Part print with two shaded views. Sizes in mm from the minimum x, y, z corner. Give positions to 0.01 mm unless a question says otherwise; leave off trailing zeros. Write each loop counter-clockwise with the first axis right and the second up, starting at its lowest first coordinate (ties: lowest second). Pieces come first, ordered by that corner, then holes. Notation, with made-up numbers: (-16.75, 46) -> (-6.75, 46) arc R27 cw to (-6.75, 64) -> close; hole circle Ø2 at (64, 45). An arc over 180 degrees is marked (long way). Answer as a JSON object with one key per item and string values.
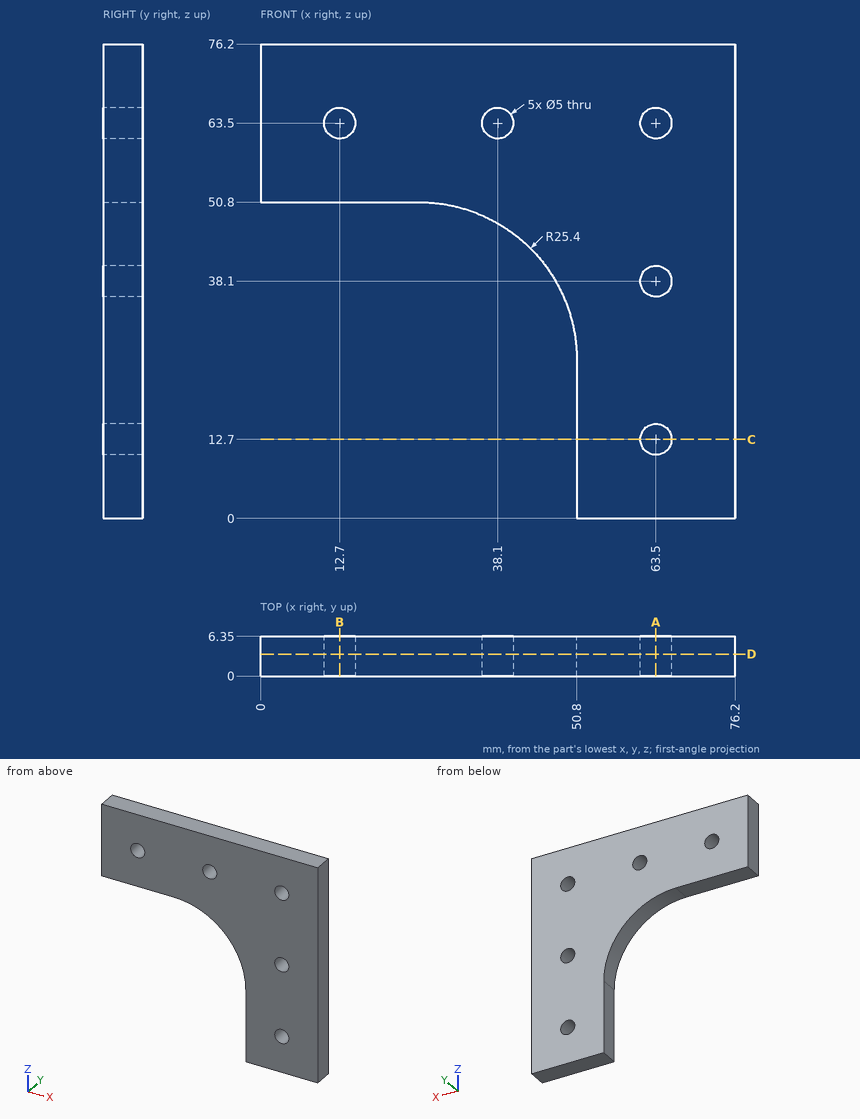
1) Slice it at B-B (x = 12.7). List the corners of the cut face in (y, z).
Model answer:
{"outline": "(0, 50.8) -> (6.35, 50.8) -> (6.35, 61) -> (0, 61) -> close; (0, 66) -> (6.35, 66) -> (6.35, 76.2) -> (0, 76.2) -> close"}
2) Slice it at D-D (y = 3.5). List the corners of the cut face in (x, z), then the cut area to 3 significant figures.
Model answer:
{"outline": "(0, 50.8) -> (25.4, 50.8) arc R25.4 cw to (50.8, 25.4) -> (50.8, 0) -> (76.2, 0) -> (76.2, 76.2) -> (0, 76.2) -> close; hole circle Ø5 at (12.7, 63.5); hole circle Ø5 at (38.1, 63.5); hole circle Ø5 at (63.5, 12.7); hole circle Ø5 at (63.5, 38.1); hole circle Ø5 at (63.5, 63.5)", "area": "3,270 mm2"}
3) Wall check: probe 1 along Z at (x, y) = (63.5, 3.25); probe 2 along Z at (x, y) = (12.7, 2.25); probe 3 along X at (y, z) = (5, 64.5). Give the ranges that are in metal, low to high.
Model answer:
{"probe 1": "z = 0 to 10.2, 15.2 to 35.6, 40.6 to 61, 66 to 76.2", "probe 2": "z = 50.8 to 61, 66 to 76.2", "probe 3": "x = 0 to 10.41, 14.99 to 35.81, 40.39 to 61.21, 65.79 to 76.2"}
4) Pin check, flat tips, straight feed: pin 1 (3 mm diameter, centred on x = 63.5, z = 12.7, fed in from +Y); pin 2 (3 mm diameter, centred on y = 3.5, z = 14, fed in from -X); pin 3 (1 mm diameter, centred on y = 3.5, z = 38.5, fed in from -X). Stop position of each tip, or through.
Model answer:
{"pin 1": "passes through", "pin 2": "stops at x = 50.8", "pin 3": "stops at x = 46.85"}
5) Slice it at C-C (z = 12.7). List the corners of the cut face in (x, y).
Model answer:
{"outline": "(50.8, 0) -> (61, 0) -> (61, 6.35) -> (50.8, 6.35) -> close; (66, 0) -> (76.2, 0) -> (76.2, 6.35) -> (66, 6.35) -> close"}
6) Slice it at A-A (x = 63.5). List the corners of the cut face in (y, z).
Model answer:
{"outline": "(0, 0) -> (6.35, 0) -> (6.35, 10.2) -> (0, 10.2) -> close; (0, 15.2) -> (6.35, 15.2) -> (6.35, 35.6) -> (0, 35.6) -> close; (0, 40.6) -> (6.35, 40.6) -> (6.35, 61) -> (0, 61) -> close; (0, 66) -> (6.35, 66) -> (6.35, 76.2) -> (0, 76.2) -> close"}
